Autodesk Inventor part; units mm, degrees
ref_plane "YZ Plane" through (0, 0, 0) normal (1, 0, 0) x (0, 1, 0)
ref_plane "XZ Plane" through (0, 0, 0) normal (0, 1, 0) x (-1, 0, 0)
ref_plane "XY Plane" through (0, 0, 0) normal (0, 0, 1) x (1, 0, 0)
sketch "Skizze1" plane through (0, 0, 0) normal (0, 0, 1) x (1, 0, 0)
  arc A0 (0, -3) -> (0, 3) centre (0, 0) ccw
  line L0 (0, 3) -> (-25.5, 3)
  line L1 (-25.5, 3) -> (-25.5, -3)
  line L2 (-25.5, -3) -> (0, -3)
  dimension "d0" = 3
  dimension "d1" = 25.5
extrude "Extrusion1" add sketch "Skizze1" along normal blind 1.5
sketch "Skizze3" plane through (-25.5, -3, 0) normal (-1, 0, 0) x (0, 0, 1)
  line L0 (0, 6) -> (0, 0)
  line L1 (0, 0) -> (1.5, 0)
  line L2 (1.5, 6) -> (1.5, 0)
  line L3 (0, 6) -> (1.5, 6)
  line L4 (0, 6) -> (4.5, 6)
  arc A0 (4.5, 0) -> (4.5, 6) centre (4.5, 3) ccw
  line L5 (4.5, 0) -> (0, 0)
  point P0 (0, 3)
  point P1 (7.5, 3)
  dimension "d4" = 7.5
extrude "Extrusion2" add sketch "Skizze3" along normal blind 1.5
sketch "Skizze4" plane through (0, 0, 1.5) normal (0, 0, 1) x (1, 0, 0)
  arc A0 (0, -3) -> (0, 3) centre (0, 0) ccw
hole "Bohrung1" at (0, 0, 1.5) direction (0, 0, -1) diameter 3 depth 1.5
properties part number "1 part 11"
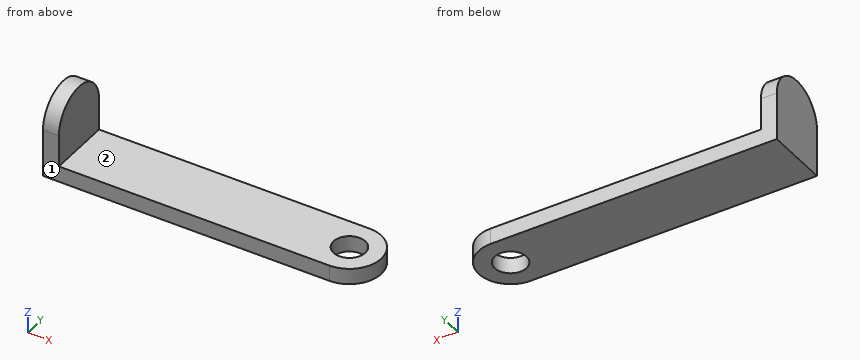
Geometry check sheet. Reference: the model listing, model coordinates, mm. Face numbers are marked on the shaded views. A direction names the side the tool comes from. Coordinates: 2 decimals unless noted, no trailing zeros. Write each loop counter-clockwise with the first axis right and the second up, starting at its lowest first coordinate (ties: lowest second). Pieces come first, ordered by that corner, then holes. Notation, with made-up numbers: M 11.25,53 L 52.25,53 A31 cw 52.25,83 Z; hole C -40,21 d8. An arc over 180 degrees is marked long. One line per item, written item: value. Start each with the question number.
(1) Tool access check on the marked faces 1 and 2. Record the directions out of +Z, -Z, +X, -X, +Y, -Y that give a thin tool (end or side, any length) a straight path to the whole face; none if there is none.
(2) Sectioned sample at C-C, the plane x = -8. Enter the section's corners in (y, z).
(3) Sectioned sample at D-D, the plane z = 5.25. Enter the section's corners in (x, y), and give its area (3 significant figures).
(4) Sectioned sample at A-A, the plane y = 0. Enter the section's corners in (x, z).
(5) Depth check by flat-ended pin: pin 1 (3 mm diameter, centred on x = -1, y = 1, fed in from +Z); pin 2 (1.5 mm diameter, centred on y = -1.5, z = 5, fed in from +X). Enter the tip coordinate at first touch or a pass-through.
(6) Scan lines: line 1 along Y through (x, z) = (0, 0.35); line 2 along X through (y, z) = (0, 0.4); line 3 along Z through (x, y) = (-24, -1.8). Record each from-to range of solid material in increasing order. Write a range as [from, to].
(7) Sectioned sample at B-B, the plane y = -1.8. Enter the section's corners in (x, z).
Filled sheet:
1. face 1: +Z, -Z, +X, -X, -Y
1. face 2: +Z, +X, +Y, -Y
2. outline: M -3,0 L 3,0 L 3,1.5 L -3,1.5 Z
3. outline: M -27,-2.9 L -25.5,-2.9 L -25.5,2.9 L -27,2.9 Z
3. area: 8.71 mm²
4. outline: M -27,0 L -1.5,0 L -1.5,1.5 L -25.5,1.5 L -25.5,7.5 L -27,7.5 Z; M 1.5,0 L 3,0 L 3,1.5 L 1.5,1.5 Z
5. pin 1: z = 1.5
5. pin 2: x = -25.5
6. line 1: [-3, -1.5], [1.5, 3]
6. line 2: [-27, -1.5], [1.5, 3]
6. line 3: [0, 1.5]
7. outline: M -27,0 L 2.4,0 L 2.4,1.5 L -25.5,1.5 L -25.5,6.9 L -27,6.9 Z
